Source: CAD feature listing. Evaluate the final solid. Frame: model axes, mm. A direction names the side the tool comes from. Coordinates: 2 decimals unless noted, no trailing zeros. Order: outer loops, then holes, each group sorted by start corner. A loop starts at its lowest first (then second) coordinate and runs counter-clockwise, first axis right, second up. Notation, with made-up numbers: (12, -14) - (37, -14) arc R10 cw to (37, -4) - close; hole circle Ø4 at (27, 79.25). An arc over 180 degrees is marked (long way). One line per question, with ' | ' between items. Start each with the question number.
(1) Access query for faces 1 (the flat face through (-2, 5.9, 5)), 2 (the flat face through (0, -7.4, 4)). Directions: +Z, -Z, +X, -X, +Y, -Y. A direction counts if a zero-diameter tool reaches every point of the face in a straight line with its end or side. Return the directions, or none.
(2) Line query: line 1 along X through (y, z) = (-3, 3.25); line 2 along Y through (x, z) = (-0.75, 4); line 3 along X through (y, z) = (0.25, 5.5). Output: solid intervals per line, ascending.
(3) Section A-A (y = -1.5). Return the cut outline in (x, z), then the cut area to 3 significant figures.
from build123d import *

# Parameters (mm, degrees)
F3_W     = 8.7
F3_H     = 11.8
F3_W_2   = 2.55
F3_W_3   = 4.75
F4_DEPTH = 3
F5_DEPTH = 7.75
F6_R     = 0.75
F7_DEPTH = 0.75
F8_R     = 0.7242640687
F9_DEPTH = 7.75


# Not quite as in the source:
# - a feature names something its author has since deleted; it is built from what else it names


with BuildPart() as f4:
    # F3 (on Top) → F4 (new body)
    with BuildSketch(Plane.XY):
        with Locations((3.65, 0)):
            Rectangle(F3_W, F3_H)
        with Locations((-1.975, 0)):
            Rectangle(F3_W_2, F3_H)
        with Locations((-5.625, 0)):
            Rectangle(F3_W_3, F3_H)
    extrude(amount=F4_DEPTH)

    # F3 (on Top) → F5 (join)
    with BuildSketch(Plane.XY):
        with Locations((3.65, 0)):
            Rectangle(F3_W, F3_H)
        Polygon((8, -7.4), (8, -5.9), (-0.7, -5.9), (-3.25, -5.9), (-8, -5.9), (-8, -7.4), align=None)
        Polygon((-0.7, 5.9), (8, 5.9), (8, 7.4), (-8, 7.4), (-8, 5.9), (-3.25, 5.9), align=None)
    extrude(amount=F5_DEPTH)

    # F6 (on face) → F7 (join)
    with BuildSketch(Plane(origin=(-0.7, 0, 0), x_dir=(0, -1, 0), z_dir=(-1, 0, 0))):
        with Locations((0, 5.75)):
            Circle(F6_R)
    extrude(amount=F7_DEPTH)

    # F8
    f8_edges = [f4.edges().sort_by_distance(p)[0] for p in [
        (-1.45, 0.75, 5.75),
    ]]
    fillet(f8_edges, radius=F8_R)

    # F3 (on Top) → F9 (join)
    with BuildSketch(Plane.XY):
        with Locations((-5.625, 0)):
            Rectangle(F3_W_3, F3_H)
    extrude(amount=F9_DEPTH)


solid = f4.part
Response values:
1) face 1: +Z | face 2: +Z, -Z, +X, -X, -Y
2) line 1: x = -8 to -3.25, -0.7 to 8 | line 2: y = -7.4 to -5.9, 5.9 to 7.4 | line 3: x = -8 to -3.25, -1.37 to 8
3) outline: (-8, 0) - (8, 0) - (8, 7.75) - (-0.7, 7.75) - (-0.7, 3) - (-3.25, 3) - (-3.25, 7.75) - (-8, 7.75) - close | area: 112 mm²
